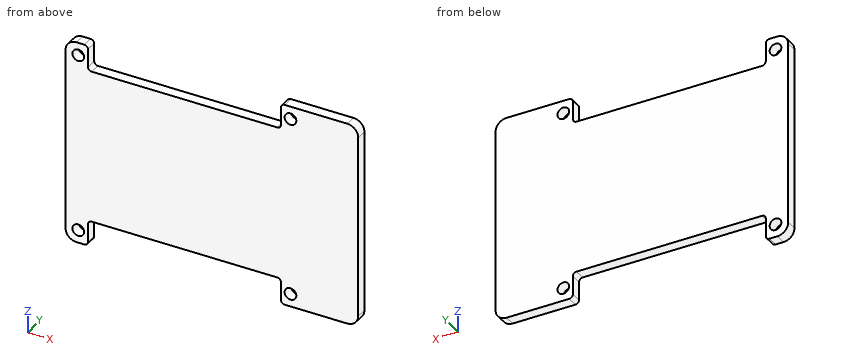
```python
from build123d import *

# Parameters (mm, degrees)
SKETCH_1_R      = 1.6
EXTRUDE_1_DEPTH = 3


with BuildPart() as part:
    # 草图1 → 凸台-拉伸1 (new body)
    with BuildSketch(Plane(origin=(0, 0, 0), x_dir=(1, 0, 0), z_dir=(0, 1, 0))):
        with BuildLine():
            Line((-21.134628196, 23.389975432), (-21.134628196, 18.377736005))
            ThreePointArc((-21.134628196, 18.377736005), (-21.427521415, 17.670629223), (-22.134628196, 17.377736005))
            Line((-22.134628196, 17.377736005), (-72.874730915, 17.377736005))
            ThreePointArc((-72.874730915, 17.377736005), (-73.581837696, 17.670629223), (-73.874730915, 18.377736005))
            Line((-73.874730915, 18.377736005), (-73.874730915, 23.389975432))
            ThreePointArc((-73.874730915, 23.389975432), (-74.167624134, 24.097082213), (-74.874730915, 24.389975432))
            Line((-74.874730915, 24.389975432), (-77.021723127, 24.389975432))
            ThreePointArc((-77.021723127, 24.389975432), (-79.134066788, 23.515014039), (-80.009028181, 21.402670377))
            Line((-80.009028181, 21.402670377), (-80.009028181, -28.604431477))
            ThreePointArc((-80.009028181, -28.604431477), (-79.134066788, -30.716775138), (-77.021723127, -31.591736531))
            Line((-77.021723127, -31.591736531), (-74.874730915, -31.591736531))
            ThreePointArc((-74.874730915, -31.591736531), (-74.167624134, -31.298843313), (-73.874730915, -30.591736531))
            Line((-73.874730915, -30.591736531), (-73.874730915, -25.64502865))
            ThreePointArc((-73.874730915, -25.64502865), (-73.581837696, -24.937921869), (-72.874730915, -24.64502865))
            Line((-72.874730915, -24.64502865), (-22.134628196, -24.64502865))
            ThreePointArc((-22.134628196, -24.64502865), (-21.427521415, -24.937921869), (-21.134628196, -25.64502865))
            Line((-21.134628196, -25.64502865), (-21.134628196, -30.591736531))
            ThreePointArc((-21.134628196, -30.591736531), (-20.841734977, -31.298843313), (-20.134628196, -31.591736531))
            Line((-20.134628196, -31.591736531), (-3.009028181, -31.591736531))
            ThreePointArc((-3.009028181, -31.591736531), (-0.887707838, -30.713056875), (-0.009028181, -28.591736531))
            Line((-0.009028181, -28.591736531), (-0.009028181, -21.760486998))
            Line((-0.009028181, -21.760486998), (-0.009028181, 21.389975432))
            ThreePointArc((-0.009028181, 21.389975432), (-0.887707838, 23.511295776), (-3.009028181, 24.389975432))
            Line((-3.009028181, 24.389975432), (-20.134628196, 24.389975432))
            ThreePointArc((-20.134628196, 24.389975432), (-20.841734977, 24.097082213), (-21.134628196, 23.389975432))
        make_face()
        with Locations(Location((-76.52848462, 20.886724226, 0), (0, 0, 270))):
            Circle(SKETCH_1_R, mode=Mode.SUBTRACT)
        with Locations(Location((-18.52858622, 20.886597225, 0), (0, 0, 270))):
            Circle(SKETCH_1_R, mode=Mode.SUBTRACT)
        with Locations(Location((-18.52833222, -28.113656775, 0), (0, 0, 270))):
            Circle(SKETCH_1_R, mode=Mode.SUBTRACT)
        with Locations(Location((-76.52833222, -28.113529775, 0), (0, 0, 270))):
            Circle(SKETCH_1_R, mode=Mode.SUBTRACT)
    extrude(amount=EXTRUDE_1_DEPTH)


solid = part.part
```
Work out the finished part from the listing and answer in its coordinate system (mm). Coordinates: 2 decimals unless noted, no trailing zeros. Write each loop counter-clockwise with the first axis right and the second up, starting at its lowest first coordinate (ties: lowest second). Pieces come first, ordered by that corner, then holes.
Q1. Find the intervals of material crossed by line 1 (X direction, y = 2.7, z = 25.5); line 2 (Z direction, x = -43, y = 0.35); line 3 (Z direction, x = -73.5, y = 0.2), in increasing order.
Q2. A cutting plane is placed at B-B, the plane x = -43. Give the vertices of the cut face in (y, z).
Q3. A cutting plane is placed at A-A, the plane y = 1.6. Give the vertices of the cut face in (x, z), then the cut area to 3 significant figures.
Q4. This flat-tipped pin is pushed along its axis until it touches: pin 1 Ø1.9 at (x, z) = (-18.53, 28.11) entering from +Y. Where does it stop, or does it pass through?
Findings below:
1. line 1: x = -80.01 to -73.86, -21.15 to -0.01
1. line 2: z = -17.38 to 24.65
1. line 3: z = -17.6 to 24.86
2. outline: (0, -17.38) - (3, -17.38) - (3, 24.65) - (0, 24.65) - close
3. outline: (-80.01, -21.4) arc R2.99 ccw to (-77.02, -24.39) - (-74.87, -24.39) arc R1 ccw to (-73.87, -23.39) - (-73.87, -18.38) arc R1 cw to (-72.87, -17.38) - (-22.13, -17.38) arc R1 cw to (-21.13, -18.38) - (-21.13, -23.39) arc R1 ccw to (-20.13, -24.39) - (-3.01, -24.39) arc R3 ccw to (-0.01, -21.39) - (-0.01, 28.59) arc R3 ccw to (-3.01, 31.59) - (-20.13, 31.59) arc R1 ccw to (-21.13, 30.59) - (-21.13, 25.65) arc R1 cw to (-22.13, 24.65) - (-72.87, 24.65) arc R1 cw to (-73.87, 25.65) - (-73.87, 30.59) arc R1 ccw to (-74.87, 31.59) - (-77.02, 31.59) arc R2.99 ccw to (-80.01, 28.6) - close; hole circle Ø3.2 at (-76.53, -20.89); hole circle Ø3.2 at (-76.53, 28.11); hole circle Ø3.2 at (-18.53, -20.89); hole circle Ø3.2 at (-18.53, 28.11)
3. area: 3,700 mm2
4. pin 1: passes through
